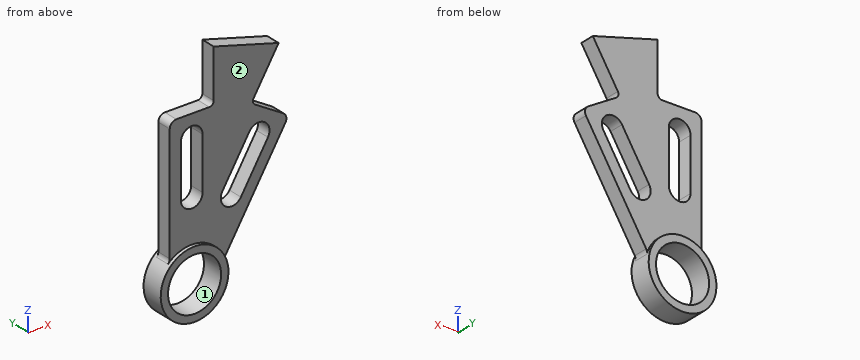
```python
from build123d import *

# Parameters (mm, degrees)
SKETCH1_R             = 14.6812
SKETCH1_R_2           = 11.5062
BEARING_EXTRUDE_DEPTH = 4.7625
BOSS_EXTRUDE2_DEPTH   = 3.175
FILLET1_R             = 2.54
FILLET2_R             = 1.905
FILLET3_R             = 2.8575


with BuildPart() as part:
    # Sketch1 → Bearing extrude (new, symmetric)
    with BuildSketch(Plane(origin=(0, 0, 0), x_dir=(1, 0, 0), z_dir=(0, 1, 0))):
        with Locations(Location((0, 0, 0), (0, 0, 90))):
            Circle(SKETCH1_R)
        with Locations(Location((0, 0, 0), (0, 0, 90))):
            Circle(SKETCH1_R_2, mode=Mode.SUBTRACT)
    extrude(amount=BEARING_EXTRUDE_DEPTH, both=True)

    # Sketch1<5> → Boss-Extrude2 (add, symmetric)
    with BuildSketch(Plane(origin=(0, 0, 0), x_dir=(1, 0, 0), z_dir=(0, 1, 0))):
        with BuildLine():
            Line((-9.525, -11.171929486), (-9.525, -65.4812))
            Line((-9.525, -65.4812), (9.525, -65.4812))
            Line((9.525, -65.4812), (9.525, -88.3412))
            Line((9.525, -88.3412), (37.653512805, -80.480471022))
            Line((37.653512805, -80.480471022), (25.802250815, -60.932397223))
            Line((25.802250815, -60.932397223), (33.947281565, -55.994371394))
            Line((33.947281565, -55.994371394), (42.092312315, -51.056345565))
            Line((42.092312315, -51.056345565), (13.936870788, -4.615329467))
            ThreePointArc((13.936870788, -4.615329467), (3.951379748, -14.13945655), (-9.525, -11.171929486))
        make_face()
        with BuildLine():
            ThreePointArc((4.699, -55.9562), (0, -60.6552), (-4.699, -55.9562))
            Line((-4.699, -55.9562), (-4.699, -33.3502))
            ThreePointArc((-4.699, -33.3502), (0, -28.6512), (4.699, -33.3502))
            Line((4.699, -33.3502), (4.699, -55.9562))
        make_face(mode=Mode.SUBTRACT)
        with BuildLine():
            ThreePointArc((33.027470906, -45.413247902), (33.573140629, -48.968070141), (31.445348478, -51.867555814))
            ThreePointArc((31.445348478, -51.867555814), (27.890526239, -52.413225537), (24.991040566, -50.285433386))
            Line((24.991040566, -50.285433386), (13.271459266, -30.954560407))
            ThreePointArc((13.271459266, -30.954560407), (14.853581693, -24.500252495), (21.307889605, -26.082374923))
            Line((21.307889605, -26.082374923), (33.027470906, -45.413247902))
        make_face(mode=Mode.SUBTRACT)
    extrude(amount=BOSS_EXTRUDE2_DEPTH, both=True)

    # Fillet1
    fillet1_edges = [part.edges().sort_by_distance(p)[0] for p in [
        (13.936870788, 0, 4.615329467),
        (-9.525, 0, 11.171929486),
    ]]
    fillet(fillet1_edges, radius=FILLET1_R)

    # Fillet2
    fillet2_edges = [part.edges().sort_by_distance(p)[0] for p in [
        (25.802250815, 0, 60.932397223),
        (9.525, 0, 65.4812),
    ]]
    fillet(fillet2_edges, radius=FILLET2_R)

    # Fillet3
    fillet3_edges = [part.edges().sort_by_distance(p)[0] for p in [
        (42.092312315, 0, 51.056345565),
        (-9.525, 0, 65.4812),
    ]]
    fillet(fillet3_edges, radius=FILLET3_R)


solid = part.part
```
Could you check a few things on this model? Use its own coordinates, in mm. Face numbers are marked on the shaded views. Give positions to 0.01 mm unless a question says otherwise; leave off trailing zeros. Loops run counter-clockwise (first coordinate to the right, second up) from the corner with the lowest first, then second, coordinate; pieces in that order, holes last. Notation, with made-up numbers: (52.25, -8.5) - (63.25, -8.5) arc R23 cw to (63.25, 0.5) - close; hole circle Ø11 at (5.25, -18.75). An arc over 180 degrees is marked (long way). Answer in a Markdown table with one row per item. Add a question column.
Q1. Please list where these lines run through material, in increasing order: L1, parallel to X at y = -1, z = 0; L2, parallel to Y at x = 15.5, z = 63 (3 decimals); L3, parallel to Z at x = 7.5, y = -2.25. Write a range as from..to.
Q2. If we section it at A-A (z = 0): List the corners of the cut face in (x, y) for me.
Q3. If we section it at B-B (x = 0): List the corners of the cut face in (y, z) for me (1 decimal).
Q4. We'd pull the mould along Z, two halves only. Please class the marked faces 1 and 2: +Z half, -Z half, draft (parallel to the pull), parting line (faces both ways), or undercut.
Q5. If we section it at C-C (x = 36.5): List the corners of the cut face in (y, z) for me (3 decimals), plus the area to 3 significant figures.
Q6. For pin 1 (1.5 mm diameter, centred on x = 30.5, y = -1.5, fed in from +Z); pin 2 (3 mm diameter, centred on x = 25.5, y = 2.5, fed in from +Z); pin 3 (5 mm diameter, centred on y = -3.5, z = 44, fed in from +X), each with a flat end and sliding along its axis, tell me the tip position at first contact or that it passes through.
Q7. If we section it at D-D (y = -1): List the corners of the cut face in (x, z) for me (1 decimal).
The answers:
| question | item | result |
|---|---|---|
| 1 | L1 | x = -14.68..-11.51, 11.51..14.68 |
| 1 | L2 | y = -3.175..3.175 |
| 1 | L3 | z = -12.62..-8.73, 8.73..65.48 |
| 2 | outline | (-14.68, -4.76) - (-11.51, -4.76) - (-11.51, 4.76) - (-14.68, 4.76) - close; (11.51, -4.76) - (14.68, -4.76) - (14.68, 4.76) - (11.51, 4.76) - close |
| 3 | outline | (-4.8, -14.7) - (4.8, -14.7) - (4.8, -11.5) - (-4.8, -11.5) - close; (-4.8, 11.5) - (4.8, 11.5) - (4.8, 14.7) - (3.2, 14.7) - (3.2, 28.7) - (-3.2, 28.7) - (-3.2, 14.7) - (-4.8, 14.7) - close; (-3.2, 60.7) - (3.2, 60.7) - (3.2, 65.5) - (-3.2, 65.5) - close |
| 4 | face 1 | undercut |
| 4 | face 2 | draft |
| 5 | outline | (-3.175, 41.832) - (3.175, 41.832) - (3.175, 54.447) - (-3.175, 54.447) - close; (-3.175, 78.578) - (3.175, 78.578) - (3.175, 80.803) - (-3.175, 80.803) - close |
| 5 | area | 94.2 mm^2 |
| 6 | pin 1 | stops at z = 82.69 |
| 6 | pin 2 | stops at z = 84.3 |
| 6 | pin 3 | stops at x = 39.32 |
| 7 | outline | (-10.3, 10.5) arc R14.7 ccw (long way) to (14.2, 3.6) arc R2.5 cw to (14.5, 5.6) - (40.6, 48.6) arc R2.9 ccw to (39.6, 52.5) - (27.4, 59.9) arc R1.9 cw to (26.8, 62.6) - (37.7, 80.5) - (9.5, 88.3) - (9.5, 67.4) arc R1.9 cw to (7.6, 65.5) - (-6.7, 65.5) arc R2.9 ccw to (-9.5, 62.6) - (-9.5, 12.3) arc R2.5 cw to start; hole circle Ø23 at (0, 0); hole (-4.7, 33.4) arc R4.7 ccw to (4.7, 33.4) - (4.7, 56) arc R4.7 ccw to (-4.7, 56) - close; hole (13.3, 31) arc R4.7 ccw to (21.3, 26.1) - (33, 45.4) arc R4.7 ccw to (25, 50.3) - close |
